from build123d import *

# Parameters (mm, degrees)
IZIM1_W                     = 70
IZIM1_H                     = 40
Y_KSEKLIK_EKSTR_ZYON2_DEPTH = 25
IZIM2_W                     = 35
IZIM2_H                     = 20
KES_EKSTR_ZYON2_DEPTH       = 67
IZIM3_W                     = 70
IZIM3_H                     = 40
KES_EKSTR_ZYON3_DEPTH       = 3
IZIM4_RX                    = 26
IZIM4_RY                    = 10
Y_KSEKLIK_EKSTR_ZYON3_DEPTH = 2
IZIM5_R                     = 1.5
KES_EKSTR_ZYON5_DEPTH       = 16


with BuildPart() as part:
    # Çizim1 → Yükseklik-Ekstrüzyon2 (new body)
    with BuildSketch(Plane(origin=(0, 0, 0), x_dir=(1, 0, 0), z_dir=(0, 1, 0))):
        with Locations((-2.232631088, 6.981597522)):
            Rectangle(IZIM1_W, IZIM1_H)
    extrude(amount=Y_KSEKLIK_EKSTR_ZYON2_DEPTH)

    # Çizim2 → Kes-Ekstrüzyon2 (cut)
    with BuildSketch(Plane.ZY.offset(37.232631088)):
        with Locations((-6.981597522, 12.5)):
            Rectangle(IZIM2_W, IZIM2_H)
    extrude(amount=-KES_EKSTR_ZYON2_DEPTH, mode=Mode.SUBTRACT)

    # Çizim3 → Kes-Ekstrüzyon3 (cut)
    with BuildSketch(Plane(origin=(0, 25, 0), x_dir=(1, 0, 0), z_dir=(0, 1, 0))):
        with Locations((-2.232631088, 6.981597522)):
            Rectangle(IZIM3_W, IZIM3_H)
    extrude(amount=-KES_EKSTR_ZYON3_DEPTH, mode=Mode.SUBTRACT)

    # Çizim4 → Yükseklik-Ekstrüzyon3 (add)
    with BuildSketch(Plane.XZ):
        with Locations(Location((-2.232631088, -6.981597522), (0, 0, 90))):
            Ellipse(IZIM4_RX, IZIM4_RY)
    extrude(amount=-Y_KSEKLIK_EKSTR_ZYON3_DEPTH)

    # Çizim5 → Kes-Ekstrüzyon5 (cut)
    with BuildSketch(Plane(origin=(0, 2, 0), x_dir=(1, 0, 0), z_dir=(0, 1, 0))):
        with Locations((-2.232631088, -16.518402478)):
            Circle(IZIM5_R)
        with Locations((-2.232631088, 30.481597522)):
            Circle(IZIM5_R)
    extrude(amount=-KES_EKSTR_ZYON5_DEPTH, mode=Mode.SUBTRACT)


solid = part.part
Can you work these out from the model? Positions are in its coordinate system, mm. A direction names the side the tool comes from. Give positions to 0.01 mm unless a question says otherwise; leave off trailing zeros. Loops run counter-clockwise (first coordinate to the right, second up) from the corner with the lowest first, then second, coordinate; pieces in that order, holes last. Notation, with made-up numbers: M 16,85 L 30,85 A15 cw 30,97 Z; hole C 69,-37 d5. An arc over 180 degrees is marked long. One line per item, written item: value. Start each with the question number.
1) Thinking about a two-plate mould opening in Z: for faces 5 (the face through (-3, 11, -26.982)), 6 (the face through (29.767, 12, -7)), 7 (the face through (-3, 0, -7)), which applies, +Z half, -Z half, draft (parallel to the pull), parting line (faces both ways), or undercut?
2) If we section it at C-C, the plane z = 6: Write out the boundary of the cut face in (x, y), and give its area (4 significant figures).
3) If we section it at A-A, the plane y = 13.25: Write out the boundary of the cut face in (x, z).
4) I'm going to push flat-ended pins straight in: pin 1 (12 mm diameter, centred on x = 9, y = 18, fed in from +Z); pin 2 (3 mm diameter, centred on x = -7.5, y = 16.5, fed in from -Z); pin 3 (17.5 mm diameter, centred on x = -0.5, z = -11.5, fed in from +Y). Where does each tip first touch, or does it pass through?
5) On a 3-axis mill with a long thin cutter (end or side, diameter ignored), from which of +Z, -Z, +X, -X, +Y, -Y can I reach the whole of each face in a straight line? I mean faces 1 (the face through (-37.233, 2, -7)), 2 (the face through (-2.3, 2, 14.6)), 3 (the face through (-2.3, 2, -28.7)), 4 (the face through (-4, 2.5, -7)). Say none if no direction works.
6) If I drill on line 1 (Z direction, x = -27, y = 10.75); line 2 (Y direction, x = 29.5, z = -8); line 3 (X direction, y = 17, z = 8), over which ranges is the centre line in solid material (lowest first)? Write a range as [from, to].
7) If we section it at B-B, the plane x = -28: Write out the boundary of the cut face in (y, z), and give its area (4 significant figures).
Completed:
1. face 5: -Z half
1. face 6: undercut
1. face 7: draft
2. outline: M -37.23,0 L 32.77,0 L 32.77,22 L 29.77,22 L 29.77,2.5 L -37.23,2.5 Z
2. area: 233.5 mm^2
3. outline: M -37.23,-26.98 L 32.77,-26.98 L 32.77,13.02 L -37.23,13.02 L -37.23,10.52 L 29.77,10.52 L 29.77,-24.48 L -37.23,-24.48 Z
4. pin 1: stops at z = 13.02
4. pin 2: stops at z = -26.98
4. pin 3: stops at y = 2.5
5. face 1: +Z, -Z, -X, +Y, -Y
5. face 2: +Z, +X, -X, +Y
5. face 3: -Z, +X, -X, +Y
5. face 4: -X, +Y
6. line 1: z = [-26.98, -24.48], [10.52, 13.02]
6. line 2: y = [0, 2.5]
6. line 3: x = [29.77, 32.77]
7. outline: M 0,-26.98 L 22,-26.98 L 22,-24.48 L 2.5,-24.48 L 2.5,10.52 L 22,10.52 L 22,13.02 L 0,13.02 Z
7. area: 197.5 mm^2
